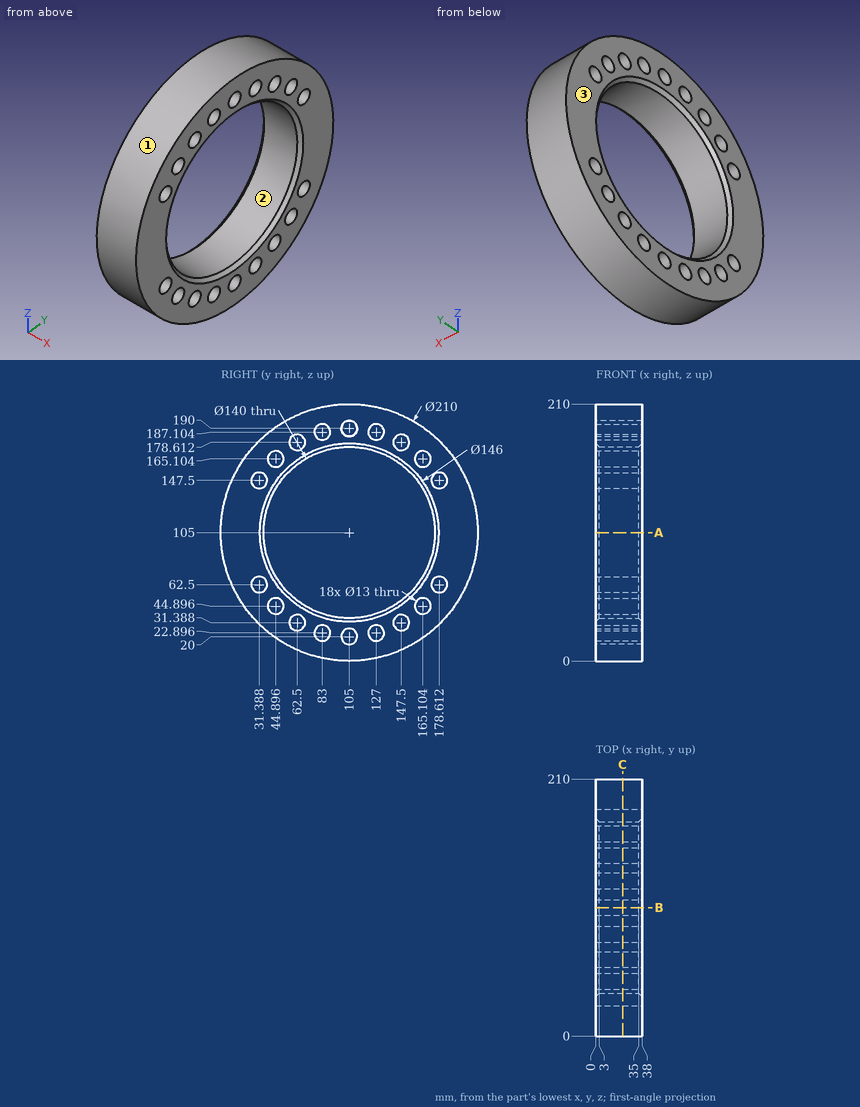
Part print with two shaded views. Sizes in mm from the minimum x, y, z corner. Round coordinates to 2 decimals unless told otherwise and drop trailing zeros. Write each loop counter-clockwise with the first axis right and the second up, starting at its lowest first coordinate (ties: lowest second). Pieces come first, ordered by that corner, then holes. Notation, with made-up numbers: (44, -25.75) -> (86, -25.75) arc R9 ccw to (86, -16.75) -> close; hole circle Ø7 at (-37, 40). An arc over 180 degrees is marked (long way). Use one line per item in the form item = value.
Q1. Drop flat-ended pins along their axis: P1, Ø11.5, axis at y = 165.1, z = 44.9, coming from the +X side; P2, Ø4, axis at x = 9.5, z = 185, coming from the +Y side; P3, Ø2, axis at x = 22.5, z = 80, coming from the -Y side; P4, Ø5, axis at x = 19.5, y = 122.5, coming from the +Z side. Give the stop position or say it passes through.
Conclusion:
P1 = through
P2 = 175.29
P3 = 2.78
P4 = 208.92
Q2. Band-saw the part on C-C, the plane x = 22. State how many separate pieces and enclosed holes the cut face has, then the cut area to 3 significant figures.
Conclusion:
separate_pieces = 1
enclosed_holes = 19
area = 16,900 mm²
Q3. Band-saw the part on B-B, the plane y = 105. Write the cut outline in (x, z), then the cut area to 3 significant figures.
Conclusion:
outline = (0, 0) -> (38, 0) -> (38, 13.5) -> (0, 13.5) -> close; (0, 26.5) -> (38, 26.5) -> (38, 32) -> (35, 35) -> (3, 35) -> (0, 32) -> close; (0, 178) -> (3, 175) -> (35, 175) -> (38, 178) -> (38, 183.5) -> (0, 183.5) -> close; (0, 196.5) -> (38, 196.5) -> (38, 210) -> (0, 210) -> close
area = 1,650 mm²
Q4. Drill centre lines: L1, parallel to Z at x = 6, y = 178; L2, parallel to Z at x = 35, y = 106 (1 decimal); L3, parallel to Y at x = 20, z = 150. Where is each one in solid material? Low to high.
Conclusion:
L1 = 29.53 to 56.03, 68.97 to 141.03, 153.97 to 180.47
L2 = 0 to 13.6, 26.4 to 35, 175 to 183.6, 196.4 to 210
L3 = 10.13 to 25.39, 37.39 to 51.38, 158.62 to 172.61, 184.61 to 199.87
Q5. Band-saw the part on A-A, the plane z = 105. Write the cut outline in (x, y).
Conclusion:
outline = (0, 0) -> (38, 0) -> (38, 32) -> (35, 35) -> (3, 35) -> (0, 32) -> close; (0, 178) -> (3, 175) -> (35, 175) -> (38, 178) -> (38, 210) -> (0, 210) -> close
Q6. Two-plate mould, pull along Z, no slides. Class the marked faces 1, 2 and 3: released by +Z, released by -Z, zero draft, split by the parting line, or undercut.
Conclusion:
face_1 = split by the parting line
face_2 = undercut
face_3 = zero draft
